from build123d import *

# Parameters (mm, degrees)
SKETCH1_R               = 9
BOSS_EXTRUDE1_DEPTH     = 20
CUT_EXTRUDE1_DEPTH      = 24.706539182
CUT_EXTRUDE1_DEPTH_BACK = 24.706539182
SKETCH2_W               = 10
SKETCH2_H               = 10
BOSS_EXTRUDE2_START     = 10
BOSS_EXTRUDE2_DEPTH     = 10
CUT_EXTRUDE2_DEPTH      = 8
CUT_EXTRUDE2_DEPTH_BACK = 24.706539182
SKETCH4_R               = 1.5
FILLET1_R               = 10
CUT_EXTRUDE3_DEPTH      = 24.706539343
CUT_EXTRUDE3_DEPTH_BACK = 24.706539343
SKETCH6_R               = 0.625
CUT_EXTRUDE4_DEPTH      = 32
CUT_EXTRUDE5_REACH      = 25.707
SKETCH7_W               = 3
SKETCH7_H               = 2
SKETCH8_R               = 0.9
CUT_EXTRUDE6_DEPTH      = 5


with BuildPart() as part:
    # Sketch1 → Boss-Extrude1 (new body)
    with BuildSketch(Plane.XY):
        Circle(SKETCH1_R)
    extrude(amount=-BOSS_EXTRUDE1_DEPTH)

    # Sketch2 → Cut-Extrude1 (cut, two sides: drawn at the far end of the back side and taken through both)
    with BuildSketch(Plane(origin=(0, 0, 0), x_dir=(1, 0, 0), z_dir=(0, 1, 0)).offset(-CUT_EXTRUDE1_DEPTH_BACK)):
        with Locations((0, 15)):
            Rectangle(SKETCH2_W, SKETCH2_H)
    extrude(amount=CUT_EXTRUDE1_DEPTH + CUT_EXTRUDE1_DEPTH_BACK, mode=Mode.SUBTRACT)

    # Sketch3 → Boss-Extrude2 (add)
    with BuildSketch(Plane.XY.offset(BOSS_EXTRUDE2_START)):
        with BuildLine():
            Line((-4.5, 7.794228634), (-4.5, -7.794228634))
            ThreePointArc((-4.5, -7.794228634), (0, -9), (4.5, -7.794228634))
            Line((4.5, -7.794228634), (4.5, 7.794228634))
            Line((4.5, 7.794228634), (-4.5, 7.794228634))
        make_face()
    extrude(amount=-BOSS_EXTRUDE2_DEPTH)

    # Sketch4 → Cut-Extrude2 (cut, two sides: drawn at the far end of the back side and taken through both)
    with BuildSketch(Plane(origin=(0, 0, 0), x_dir=(0, 0, -1), z_dir=(1, 0, 0)).offset(-CUT_EXTRUDE2_DEPTH_BACK)):
        with Locations((-5, 0)):
            Circle(SKETCH4_R)
        with Locations((16, 0)):
            Circle(SKETCH4_R)
    extrude(amount=CUT_EXTRUDE2_DEPTH + CUT_EXTRUDE2_DEPTH_BACK, mode=Mode.SUBTRACT)

    # Fillet1
    fillet1_edges = [part.edges().sort_by_distance(p)[0] for p in [
        (0, 7.794228634, 10),
    ]]
    fillet(fillet1_edges, radius=FILLET1_R - 0.0001)  # a hair under: the kernel refuses the full size

    # Sketch5 → Cut-Extrude3 (cut, two sides: drawn at the far end of the back side and taken through both)
    with BuildSketch(Plane(origin=(0, 0, 0), x_dir=(0, 0, -1), z_dir=(1, 0, 0)).offset(-CUT_EXTRUDE3_DEPTH_BACK)):
        with BuildLine():
            Line((10, 7.483314774), (20, 7.483314774))
            Line((20, 7.483314774), (20, 0))
            ThreePointArc((20, 0), (16.031389946, 5.119910176), (10, 7.483314774))
        make_face()
    extrude(amount=CUT_EXTRUDE3_DEPTH + CUT_EXTRUDE3_DEPTH_BACK, mode=Mode.SUBTRACT)

    # Sketch6 → Cut-Extrude4 (cut)
    with BuildSketch(Plane(origin=(0, 0, -20), x_dir=(-1, 0, 0), z_dir=(0, 0, -1))):
        with Locations(Location((0, 7.5, 0), (0, 0, 28.084018699))):
            Circle(SKETCH6_R)
    extrude(amount=-CUT_EXTRUDE4_DEPTH, mode=Mode.SUBTRACT)

    # Sketch7 → Cut-Extrude5 (cut, up to next)
    with BuildSketch(Plane(origin=(0, 0, -10), x_dir=(-1, 0, 0), z_dir=(0, 0, -1)), mode=Mode.PRIVATE) as cut_extrude5_sk1:
        with Locations((0, -9)):
            Rectangle(SKETCH7_W, SKETCH7_H)
    cut_extrude5_tool1 = extrude(cut_extrude5_sk1.sketch, amount=-CUT_EXTRUDE5_REACH, mode=Mode.PRIVATE) & part.part
    add(cut_extrude5_tool1.solids().sort_by_distance((0, -9, -10))[0], mode=Mode.SUBTRACT)

    # Sketch8 → Cut-Extrude6 (cut)
    with BuildSketch(Plane(origin=(0, -8, 0), x_dir=(-1, 0, 0), z_dir=(0, -1, 0))):
        with Locations(Location((0, 0, 0), (0, 0, 90))):
            Circle(SKETCH8_R)
    extrude(amount=-CUT_EXTRUDE6_DEPTH, mode=Mode.SUBTRACT)


solid = part.part
Check sheet for the modelled part. Datum: model origin and axes. Units: mm. A direction names the side the tool comes from. Round coordinates to 2 decimals unless told otherwise and drop trailing zeros. Order: outer loops, then holes, each group sorted by start corner. A loop starts at its lowest first (then second) coordinate and runs counter-clockwise, first axis right, second up.
(1) Cross-section at C-C, the plane z = -16. Enter the section's corners in (x, y), and give its area (3 significant figures).
(2) Go/stop test with flat-tipped pins: P1, Ø0.8, axis at x = 0, y = 7.5, coming from the -Z side; P2, Ø3, axis at y = -2.5, z = -9.5, coming from the +X side; P3, Ø10, axis at x = -4, z = -12.5, coming from the +Y side; P4, Ø3, axis at x = -1, y = -2, coming from the -Z side. Record where each tip stops, or that it passes through.
(3) Draft check along Z on faces 6 (the flat face through (-1.3, -8, -0.1)), 7 (the flat face through (-7, -3, -20)), 8 (the cylindrical face through (-0.345, -5.535, -0.831)). Enter one of: pulls with the +Z half, pulls with the -Z half, needs draft (parallel to the pull), parting line crosses it, or undercut.
(4) Cross-section at D-D, the plane y = -5.25. Enter the section's corners in (x, z).
(5) Cross-section at A-A, the plane x = 0. Enter the section's corners in (y, z) (3 decimals).
(6) Cross-section at B-B, the plane z = -4. Enter the section's corners in (x, y) (3 decimals).
(7) Access from +Z, -Z, +X, -X, +Y, -Y to the whole of each face (thin tool, end or side, straight path). Record for faces 1 (the flat face through (0, -3, 0)), 2 (the flat face through (1.5, -8.4, -0.1)), 3 (the flat face through (0, 0, -10)), 4 (the flat face through (-6, 0, 0)), 5 (the flat face through (6, 0, 0)).
(8) Scan lines: probe 1 along Z at (x, y) = (-6.25, 0); probe 2 along X at (y, z) = (7.5, 0.75) (3 decimals); probe 3 along X at (y, z) = (7, 1) (3 decimals). Record each from-to range of solid material in increasing order.
Check sheet entries:
1. outline: (-8.87, -1.5) arc R9 ccw to (-5, -7.48) - (-5, -1.5) - close; (-8.87, 1.5) - (-5, 1.5) - (-5, 5.14) - (-7.39, 5.14) arc R9 ccw to start; (5, -7.48) arc R9 ccw to (7.39, 5.14) - (5, 5.14) - (5, 1.5) - (8, 1.5) - (8, -1.5) - (5, -1.5) - close
1. area: 57.1 mm2
2. P1: passes through
2. P2: stops at x = 8.94
2. P3: stops at y = 9
2. P4: stops at z = -10
3. face 6: needs draft
3. face 7: pulls with the -Z half
3. face 8: undercut
4. outline: (-7.31, -20) - (-5, -20) - (-5, -10) - (5, -10) - (5, -20) - (7.31, -20) - (7.31, 0) - (4.5, 0) - (4.5, 10) - (-4.5, 10) - (-4.5, 0) - (-7.31, 0) - close; hole circle Ø1.8 at (0, 0)
5. outline: (-8, -10) - (6.875, -10) - (6.875, 4.188) arc R10 ccw to (-2.206, 10) - (-8, 10) - (-8, 0.9) - (-3, 0.9) - (-3, -0.9) - (-8, -0.9) - close; (8.125, -10) - (9, -10) - (9, 0) - (8.125, 0) - close; hole circle Ø3 at (0, 5)
6. outline: (-1.5, -8.874) - (-1.5, -8) - (1.5, -8) - (1.5, -8.874) arc R9 ccw (long way) to start; hole circle Ø1.25 at (0, 7.5)
7. face 1: -Y
7. face 2: +Z, -Z, -Y
7. face 3: -Z, +Y, -Y
7. face 4: +Z, -X, +Y, -Y
7. face 5: +Z, +X, +Y, -Y
8. probe 1: z = -20 to -17.5, -14.5 to 0
8. probe 2: x = -4.5 to -0.625, 0.625 to 4.5
8. probe 3: x = -4.5 to -0.375, 0.375 to 4.5
